from build123d import *

# Parameters (mm, degrees)
ESQUISSE2_R             = 55
ENL_V_MAT_EXTRU_1_DEPTH = 242.016596939
TROU_TARAUD_M1010_D     = 8.5
PER_AGE16_D             = 18
PER_AGE16_DEPTH         = 90
PER_AGE16_CBORE_D       = 25
PER_AGE16_CBORE_DEPTH   = 40
PER_AGE17_D             = 18
PER_AGE17_DEPTH         = 90
PER_AGE17_CBORE_D       = 25
PER_AGE17_CBORE_DEPTH   = 40


with BuildPart() as part:
    # Esquisse1 → Révolution1 (revolve)
    with BuildSketch(Plane.XY, mode=Mode.PRIVATE) as r_volution1_sk:
        Polygon((0, 0), (0, 102.2), (-45, 102.2), (-45, 160), (-128, 160), (-128, 148.5), (-111, 148.5), (-111, 100), (-58, 100), (-58, 75), (-45, 75), (-45, 0), align=None)
    revolve(r_volution1_sk.sketch.rotate(Axis((-45, 0, 0), (1, 0, 0)), 180), axis=Axis((-45, 0, 0), (1, 0, 0)))

    # Esquisse2 → Enlèv. mat.-Extru.1 (cut, through all)
    with BuildSketch(Plane.ZY.offset(45)):
        with Locations(Location((0, 0, 0), (0, 0, 270))):
            Circle(ESQUISSE2_R)
    extrude(amount=-ENL_V_MAT_EXTRU_1_DEPTH, mode=Mode.SUBTRACT)

    # Trou taraudé M1010 (through all)
    with Locations(Plane(origin=(-111, 0, -130), x_dir=(0, -1, 0), z_dir=(-1, 0, 0))):
        with Locations((0, 0), (130, 130), (0, 260), (-130, 130)):
            Hole(TROU_TARAUD_M1010_D / 2)

    # Perçage16
    with Locations(Plane(origin=(-111, 65, -112.583302492), x_dir=(0, -1, 0), z_dir=(-1, 0, 0))):
        with Locations((0, 0), (-47.583302492, 47.583302492)):
            CounterBoreHole(PER_AGE16_D / 2, PER_AGE16_CBORE_D / 2, PER_AGE16_CBORE_DEPTH, depth=PER_AGE16_DEPTH)

    # Perçage17
    with Locations(Plane(origin=(-111, 112.844971207, 64.544654878), x_dir=(0, -1, 0), z_dir=(-1, 0, 0))):
        with Locations((0, 0), (47.582560607, 47.88673648), (178.107381807, 47.88673648), (225.386921388, 0.526916867), (225.468167625, -129.475507548), (177.582207006, -177.279256049)):
            CounterBoreHole(PER_AGE17_D / 2, PER_AGE17_CBORE_D / 2, PER_AGE17_CBORE_DEPTH, depth=PER_AGE17_DEPTH)


solid = part.part
For this review, take the finished solid that the model builds, in its own axes (mm). A direction names the side the tool comes from. Give positions to 0.01 mm unless a question says otherwise; leave off trailing zeros. Write each loop counter-clockwise with the first axis right and the second up, starting at its lowest first coordinate (ties: lowest second). Pieces come first, ordered by that corner, then holes. Notation, with made-up numbers: (72.5, -7.75) -> (92.5, -7.75) arc R33 cw to (92.5, 29.25) -> close; hole circle Ø4 at (12, -21). An arc over 180 degrees is marked (long way). Use CSV: the item, a comma, the result in double quotes.
Q1. Take a section at B-B, the plane y = 0. State how many separate pieces and enclosed holes the cut face has, then the cut area to 3 significant figures.
Conclusion:
separate pieces,"4"
enclosed holes,"0"
area,"12,100 mm2"
Q2. Take a section at A-A, the plane z = -15.5. Write out the cut boundary in (x, y), then the cut area to 3 significant figures.
Conclusion:
outline,"(-128, -159.25) -> (-45, -159.25) -> (-45, -101.02) -> (0, -101.02) -> (0, -52.77) -> (-45, -52.77) -> (-45, -73.38) -> (-58, -73.38) -> (-58, -98.79) -> (-111, -98.79) -> (-111, -147.69) -> (-128, -147.69) -> close; (-128, 147.69) -> (-111, 147.69) -> (-111, 98.79) -> (-58, 98.79) -> (-58, 73.38) -> (-45, 73.38) -> (-45, 52.77) -> (0, 52.77) -> (0, 101.02) -> (-45, 101.02) -> (-45, 159.25) -> (-128, 159.25) -> close"
area,"13,400 mm2"
Q3. Take a section at D-D, the plane y = -34. Write out the cut boundary in (x, z), then the cut area to 3 significant figures.
Conclusion:
outline,"(-128, -156.35) -> (-45, -156.35) -> (-45, -96.38) -> (0, -96.38) -> (0, -43.23) -> (-45, -43.23) -> (-45, -66.85) -> (-58, -66.85) -> (-58, -94.04) -> (-111, -94.04) -> (-111, -144.56) -> (-128, -144.56) -> close; (-128, 144.56) -> (-111, 144.56) -> (-111, 94.04) -> (-58, 94.04) -> (-58, 66.85) -> (-45, 66.85) -> (-45, 43.23) -> (0, 43.23) -> (0, 96.38) -> (-45, 96.38) -> (-45, 156.35) -> (-128, 156.35) -> close"
area,"14,100 mm2"
Q4. Tool access review of faces 1 (the face through (-22.82, 22.15, 99.77)), 2 (the face through (-71, 116, -56)), 3 (the face through (-77.538, -0.553, 134.214)): name each direction out of +Z, -Z, +X, -X, +Y, -Y from which nothing blocks a thin tool from reaching the whole face with its end or side.
Conclusion:
face 1,"+X"
face 2,"-X"
face 3,"+X, -X"
Q5. To check wall thickness, follow probe 1 along Z at (x, y) = (-88, 0); probe 2 along Z at (x, y) = (-56.5, 113); probe 3 along Z at (x, y) = (-58, -111). State the ranges of each line that lie inside material, in increasing order. Write a range as [from, to].
Conclusion:
probe 1,"[-160, -134.25], [-125.75, -100], [100, 125.75], [134.25, 160]"
probe 2,"[-113.27, -73.99], [-56.01, 55.55], [73.54, 113.27]"
probe 3,"[-115.23, -73.78], [-56.08, 56.2], [73.94, 115.23]"
Q6. Mouldability with a two-part tool opening along Y and no side actions: class faces 4 (the face through (-45, 104, -2)), 5 (the face through (-71, 57, 107)), 6 (the face through (-87.081, 159.845, -7.035)) as pulls with the +Y half, pulls with the -Y half, needs draft (parallel to the pull), parting line crosses it, or undercut.
Conclusion:
face 4,"needs draft"
face 5,"undercut"
face 6,"parting line crosses it"
Q7. For P1, Ø5, axis at y = -79.5, z = -123.5, coming from the +X side; P2, Ø8, axis at x = -101, y = -30, coming from the -Z side; P3, Ø1.5, axis at x = -65, y = -7, coming from the +Z side, all flat-tipped, find the tip position at first contact; note any pin that passes through.
Conclusion:
P1,"x = -45"
P2,"z = -157.87"
P3,"z = 159.88"
